Check sheet for the modelled part. Datum: model origin and axes. Units: mm. Face numbers are marked on the shaded views. A direction names the side the tool comes from. Round coordinates to 2 decimals unless told otherwise and drop trailing zeros. Order: outer loops, then holes, each group sorted by start corner. A loop starts at its lowest first (then second) coordinate and runs counter-clockwise, first axis right, second up. Notation, with made-up numbers: M 88,88.5 L 99,88.5 A14 cw 99,109.5 Z; hole C -12.5,40.25 d7. An arc over 180 degrees is marked long. One line per item, written item: value. Start each with the question number.
(1) Cross-section at B-B, the plane z = 5.75. Count the separate pieces of the cut face and the enclosed holes in it, and give its area (3 significant figures).
(2) Cross-section at D-D, the plane x = 4. Enter the section's corners in (y, z), and give its area (3 significant figures).
(3) Cross-section at C-C, the plane z = 2.25. Enter the section's corners in (x, y).
(4) Access from +Z, -Z, +X, -X, +Y, -Y to the whole of each face (thin tool, end or side, straight path). Record for the marked faces 5, 6 and 7.
(5) Depth check by flat-ended pin: pin 1 Ø0.8 at (y, z) = (-23, 2.5) entering from +X; pin 2 Ø3.5 at (x, y) = (20, -13.5) entering from +Z; pin 3 Ø4 at (x, z) = (21, 8) entering from -Y; pin 4 Ø2.5 at (x, y) = (22.5, -33) entering from +Z. Enter the tip coordinate at first touch or a pass-through.
(6) Thickness scan on L1, parallel to Y at x = 3, z = 3.5; L2, parallel to Y at x = 22.5, z = 0; L3, parallel to Z at x = -22.5, y = 14.5. Record the ranges inside material, lowest first.
(7) Release check for a two-part mould opening along X. For the marked faces 1, 2, 3 and 4 record: released by +X, released by -X, zero draft, split by the parting line, or undercut.
(8) Cross-section at A-A, the plane y = 33. Enter the section's corners in (x, z).
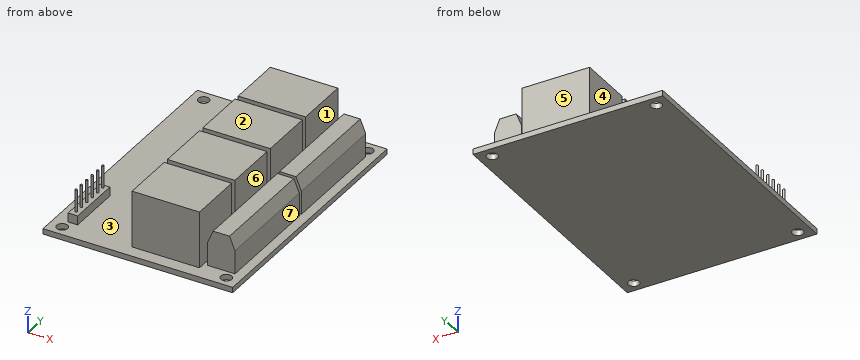
from build123d import *

# Parameters (mm, degrees)
CROQUIS1_W              = 52
CROQUIS1_H              = 72
SALIENTE_EXTRUIR1_DEPTH = 0.75
CROQUIS2_R              = 1.5
CORTAR_EXTRUIR1_DEPTH   = 1.5
CROQUIS3_W              = 18.5
CROQUIS3_H              = 15
SALIENTE_EXTRUIR2_DEPTH = 15.5
CROQUIS4_W              = 7.5
CROQUIS4_H              = 30
SALIENTE_EXTRUIR3_DEPTH = 10
CORTAR_EXTRUIR2_DEPTH   = 80
CROQUIS6_W              = 2.6
CROQUIS6_H              = 15
SALIENTE_EXTRUIR4_DEPTH = 2.5
CROQUIS7_R              = 0.3
SALIENTE_EXTRUIR5_DEPTH = 6.1


with BuildPart() as part:
    # Croquis1 → Saliente-Extruir1 (new body, symmetric)
    with BuildSketch(Plane.XY):
        Rectangle(CROQUIS1_W, CROQUIS1_H)
    extrude(amount=SALIENTE_EXTRUIR1_DEPTH, both=True)

    # Croquis2 → Cortar-Extruir1 (cut)
    with BuildSketch(Plane.XY.offset(0.75)):
        with Locations((-22.5, 33)):
            Circle(CROQUIS2_R)
        with Locations((22.5, 33)):
            Circle(CROQUIS2_R)
        with Locations((-22.5, -33)):
            Circle(CROQUIS2_R)
        with Locations((22.5, -33)):
            Circle(CROQUIS2_R)
    extrude(amount=-CORTAR_EXTRUIR1_DEPTH, mode=Mode.SUBTRACT)

    # Croquis3 → Saliente-Extruir2 (add)
    with BuildSketch(Plane.XY.offset(0.75)):
        with Locations((5.55, -24.9)):
            Rectangle(CROQUIS3_W, CROQUIS3_H)
        with Locations((5.55, -8.4)):
            Rectangle(CROQUIS3_W, CROQUIS3_H)
        with Locations((5.55, 8.1)):
            Rectangle(CROQUIS3_W, CROQUIS3_H)
        with Locations((5.55, 24.6)):
            Rectangle(CROQUIS3_W, CROQUIS3_H)
    extrude(amount=SALIENTE_EXTRUIR2_DEPTH)

    # Croquis4 → Saliente-Extruir3 (add)
    with BuildSketch(Plane.XY.offset(0.75)):
        with Locations((19.65, -15.5)):
            Rectangle(CROQUIS4_W, CROQUIS4_H)
        with Locations((19.65, 15.5)):
            Rectangle(CROQUIS4_W, CROQUIS4_H)
    extrude(amount=SALIENTE_EXTRUIR3_DEPTH)

    # Croquis5 → Cortar-Extruir2 (cut)
    with BuildSketch(Plane.XZ.offset(30.5)):
        Polygon((15.9, 10.75), (15.9, 7.15), (17.4, 10.75), align=None)
        Polygon((23.4, 10.75), (21.9, 10.75), (23.4, 7.15), align=None)
    extrude(amount=-CORTAR_EXTRUIR2_DEPTH, mode=Mode.SUBTRACT)

    # Croquis6 → Saliente-Extruir4 (add)
    with BuildSketch(Plane.XY.offset(0.75)):
        with Locations((-21.1, -22.9)):
            Rectangle(CROQUIS6_W, CROQUIS6_H)
    extrude(amount=SALIENTE_EXTRUIR4_DEPTH)

    # Croquis7 → Saliente-Extruir5 (add)
    with BuildSketch(Plane.XY.offset(3.25)):
        with Locations((-21.1, -28.9)):
            Circle(CROQUIS7_R)
        with Locations((-21.1, -26.4)):
            Circle(CROQUIS7_R)
        with Locations((-21.1, -23.9)):
            Circle(CROQUIS7_R)
        with Locations((-21.1, -21.4)):
            Circle(CROQUIS7_R)
        with Locations((-21.1, -18.9)):
            Circle(CROQUIS7_R)
        with Locations((-21.1, -16.4)):
            Circle(CROQUIS7_R)
    extrude(amount=SALIENTE_EXTRUIR5_DEPTH)


solid = part.part
Values found:
1. separate pieces: 12
1. enclosed holes: 0
1. area: 1,560 mm^2
2. outline: M -36,-0.75 L 36,-0.75 L 36,0.75 L 32.1,0.75 L 32.1,16.25 L 17.1,16.25 L 17.1,0.75 L 15.6,0.75 L 15.6,16.25 L 0.6,16.25 L 0.6,0.75 L -0.9,0.75 L -0.9,16.25 L -15.9,16.25 L -15.9,0.75 L -17.4,0.75 L -17.4,16.25 L -32.4,16.25 L -32.4,0.75 L -36,0.75 Z
2. area: 1,040 mm^2
3. outline: M -22.4,-30.4 L -19.8,-30.4 L -19.8,-15.4 L -22.4,-15.4 Z; M -3.7,-32.4 L 14.8,-32.4 L 14.8,-17.4 L -3.7,-17.4 Z; M -3.7,-15.9 L 14.8,-15.9 L 14.8,-0.9 L -3.7,-0.9 Z; M -3.7,0.6 L 14.8,0.6 L 14.8,15.6 L -3.7,15.6 Z; M -3.7,17.1 L 14.8,17.1 L 14.8,32.1 L -3.7,32.1 Z; M 15.9,-30.5 L 23.4,-30.5 L 23.4,-0.5 L 15.9,-0.5 Z; M 15.9,0.5 L 23.4,0.5 L 23.4,30.5 L 15.9,30.5 Z
4. face 5: +Z, +X, -X, +Y
4. face 6: +Z, +Y, -Y
4. face 7: +Z, +X, +Y, -Y
5. pin 1: x = 23.4
5. pin 2: z = 10.75
5. pin 3: y = -30.5
5. pin 4: through
6. L1: -32.4 to -17.4, -15.9 to -0.9, 0.6 to 15.6, 17.1 to 32.1
6. L2: -36 to -34.5, -31.5 to 31.5, 34.5 to 36
6. L3: -0.75 to 0.75
7. face 1: undercut
7. face 2: zero draft
7. face 3: undercut
7. face 4: released by -X
8. outline: M -26,-0.75 L -24,-0.75 L -24,0.75 L -26,0.75 Z; M -21,-0.75 L 21,-0.75 L 21,0.75 L -21,0.75 Z; M 24,-0.75 L 26,-0.75 L 26,0.75 L 24,0.75 Z
